Can you work these out from the model? Positions are in its coordinate system, mm. Face numbers are marked on the shaded views. A direction names the side the tool comes from. Round coordinates to 2 decimals unless told otherwise and drop trailing zeros. Loops run counter-clockwise (first coordinate to the right, second up) from the corner with the lowest first, then second, coordinate; pieces in that order, holes last. Notation, with made-up numbers: (32.5, 29.5) -> (40.5, 29.5) arc R16 cw to (40.5, 41.5) -> close; hole circle Ø5 at (17, 81.5). An arc over 180 degrees is marked (long way). Answer as a JSON object with one key per item and string values.
```python
from build123d import *

# Parameters (mm, degrees)
SKETCH1_W          = 50
SKETCH1_H          = 50
SKETCH1_W_2        = 40
SKETCH1_H_2        = 40
EXTRUDE1_DEPTH     = 50
SKETCH2_W          = 40
SKETCH2_H          = 40
CUT_EXTRUDE1_DEPTH = 50
SKETCH3_W          = 40
SKETCH3_H          = 40
CUT_EXTRUDE2_DEPTH = 10
SKETCH4_W          = 24.4
SKETCH4_H          = 40
SKETCH4_W_2        = 6.57952911
CUT_EXTRUDE3_DEPTH = 10
SKETCH5_R          = 1.016
CUT_EXTRUDE4_DEPTH = 10
SKETCH6_W          = 3
SKETCH6_H          = 12
CUT_EXTRUDE5_DEPTH = 40


with BuildPart() as part:
    # Sketch1 → Extrude1 (new body)
    with BuildSketch(Plane.XY):
        with Locations((-25, 25)):
            Rectangle(SKETCH1_W, SKETCH1_H)
        with Locations((-25, 25)):
            Rectangle(SKETCH1_W_2, SKETCH1_H_2, mode=Mode.SUBTRACT)
    extrude(amount=EXTRUDE1_DEPTH)

    # Sketch2 → Cut-Extrude1 (cut)
    with BuildSketch(Plane.XZ):
        with Locations((-25, 25)):
            Rectangle(SKETCH2_W, SKETCH2_H)
    extrude(amount=-CUT_EXTRUDE1_DEPTH, mode=Mode.SUBTRACT)

    # Sketch3 → Cut-Extrude2 (cut)
    with BuildSketch(Plane.ZY.offset(50)):
        with Locations((25, 25)):
            Rectangle(SKETCH3_W, SKETCH3_H)
    extrude(amount=-CUT_EXTRUDE2_DEPTH, mode=Mode.SUBTRACT)

    # Sketch4 → Cut-Extrude3 (cut)
    with BuildSketch(Plane(origin=(0, 0, 0), x_dir=(0, 0, -1), z_dir=(1, 0, 0))):
        with Locations((-28.77952911, 25)):
            Rectangle(SKETCH4_W, SKETCH4_H)
        with Locations((-8.289764555, 25)):
            Rectangle(SKETCH4_W_2, SKETCH4_H)
    extrude(amount=-CUT_EXTRUDE3_DEPTH, mode=Mode.SUBTRACT)

    # Sketch5 → Cut-Extrude4 (cut)
    with BuildSketch(Plane(origin=(0, 0, 0), x_dir=(0, 0, -1), z_dir=(1, 0, 0))):
        with Locations((-42.55752911, 29.616065633)):
            Circle(SKETCH5_R)
        with Locations((-42.55752911, 22.692268102)):
            Circle(SKETCH5_R)
        with Locations(Location((-15.00152911, 22.692268102, 0), (0, 0, 270))):
            Circle(SKETCH5_R)
        with Locations(Location((-15.00152911, 29.616065633, 0), (0, 0, 270))):
            Circle(SKETCH5_R)
    extrude(amount=-CUT_EXTRUDE4_DEPTH, mode=Mode.SUBTRACT)

    # Sketch6 → Cut-Extrude5 (cut)
    with BuildSketch(Plane.XY.offset(50)):
        with Locations((-3.5, 26.156065633)):
            Rectangle(SKETCH6_W, SKETCH6_H)
    extrude(amount=-CUT_EXTRUDE5_DEPTH, mode=Mode.SUBTRACT)


solid = part.part
```
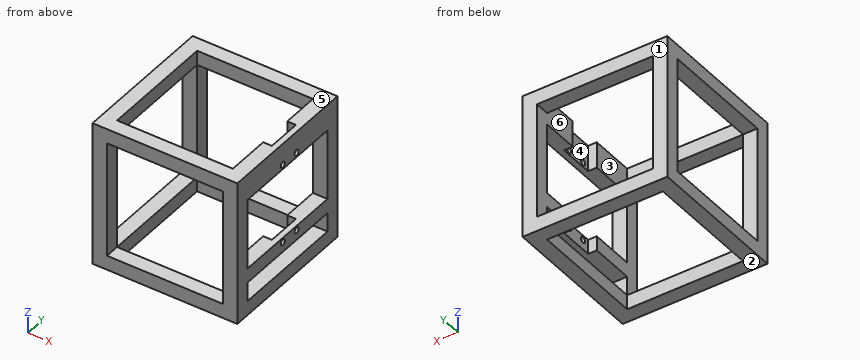
Q1. If I drill on L1, parallel to Z at x = -4, y = 10; L2, parallel to Z at x = -12.5, y = 45.5; L3, parallel to X at y = 24.5, z = 4, over which ranges is the centre line in solid material (lowest first)? Write a range as [from, to].
Determined:
{"L1": "[0, 5], [11.58, 16.58], [40.98, 50]", "L2": "[0, 5], [45, 50]", "L3": "[-50, -45], [-5, 0]"}
Q2. I want a section at A-A, the plane z = 9. Write out the boundary of the cut face in (x, y), then the cut area to 3 significant figures.
Determined:
{"outline": "(-50, 0) -> (-45, 0) -> (-45, 5) -> (-50, 5) -> close; (-50, 45) -> (-45, 45) -> (-45, 50) -> (-50, 50) -> close; (-5, 0) -> (0, 0) -> (0, 5) -> (-5, 5) -> close; (-5, 45) -> (0, 45) -> (0, 50) -> (-5, 50) -> close", "area": "100 mm²"}
Q3. On a 3-axis mill with a long thin cutter (end or side, diameter ignored), from which of +Z, -Z, +X, -X, +Y, -Y can I reach the whole of each face in a straight line? I mean the marked faces 4, 5 and 6. Say none if no direction works.
Determined:
{"face 4": "+Z", "face 5": "+Z, +X, -X, +Y, -Y", "face 6": "none"}
Q4. I'm going to push a flat-ended pin straight in: pin 1 (12 mm diameter, centred on x = -37.5, z = 30.5, fed in from -Y). Where does the tip first touch, or does it pass through?
Determined:
{"pin 1": "through"}
Q5. I want a section at C-C, the plane x = -25. Write out the boundary of the cut face in (y, z).
Determined:
{"outline": "(0, 0) -> (5, 0) -> (5, 5) -> (0, 5) -> close; (0, 45) -> (5, 45) -> (5, 50) -> (0, 50) -> close; (45, 0) -> (50, 0) -> (50, 5) -> (45, 5) -> close; (45, 45) -> (50, 45) -> (50, 50) -> (45, 50) -> close"}
Q6. I want a section at B-B, the plane y = 39. Write out the boundary of the cut face in (x, z), then the cut area to 3 significant figures.
Determined:
{"outline": "(-50, 0) -> (-45, 0) -> (-45, 5) -> (-50, 5) -> close; (-50, 45) -> (-45, 45) -> (-45, 50) -> (-50, 50) -> close; (-5, 0) -> (0, 0) -> (0, 5) -> (-5, 5) -> close; (-5, 11.58) -> (0, 11.58) -> (0, 16.58) -> (-5, 16.58) -> close; (-5, 40.98) -> (0, 40.98) -> (0, 50) -> (-5, 50) -> close", "area": "145 mm²"}
Q7. We'd pull the mould along Y, two halves only. Please class the marked faces 1, 2 and 3: pulls with the +Y half, pulls with the -Y half, needs draft (parallel to the pull), parting line crosses it, or undercut.
Determined:
{"face 1": "pulls with the +Y half", "face 2": "needs draft", "face 3": "undercut"}
